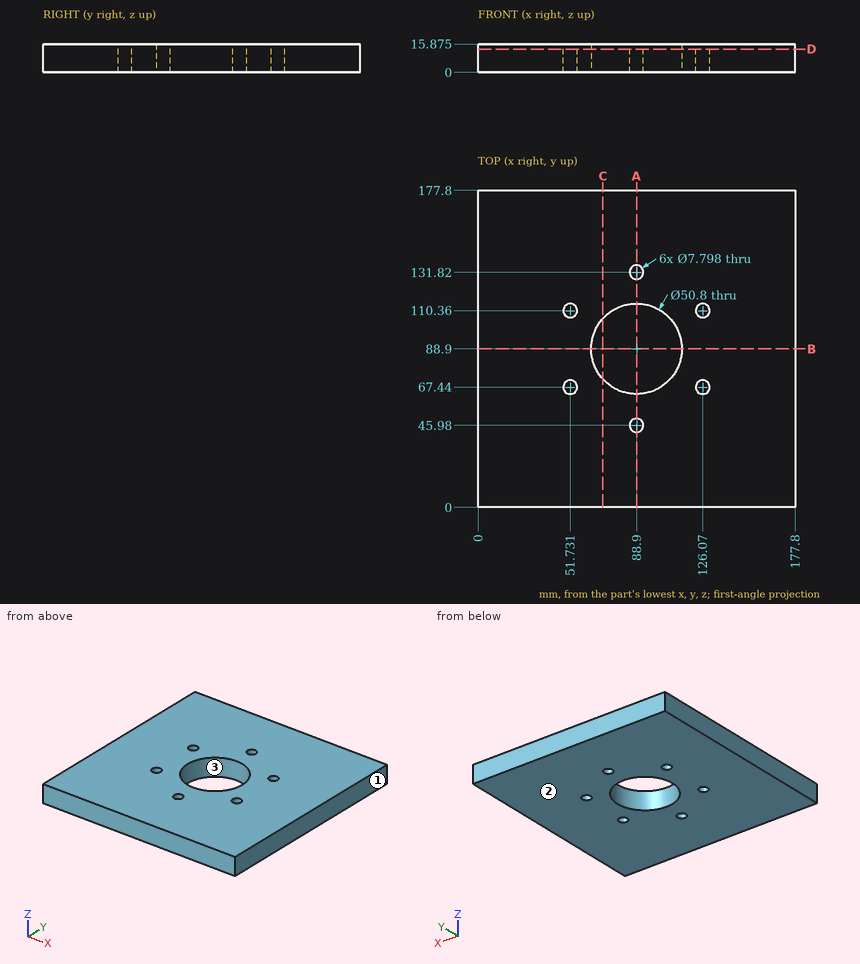
Geometry: see drawing. Coordinates: mm, zero at the bounding-box minimum. Round coordinates to 2 decimals unless told otherwise and drop trailing zeros. Loops run counter-clockwise (first coordinate to the right, second up) from the corner with the lowest first, then second, coordinate; pieces in that order, holes last. Notation, with made-up numbers: M 21.25,46.25 L 32.25,46.25 A10 ccw 32.25,64.25 Z; hole C 63.5,14 d10. An arc over 180 degrees is marked long. Use a Markdown table: item, result. Add a question column.
1. Contact query for flat-ended pins moving along their axis: pin 1 (10 mm diameter, centred on x = 126, y = 121, fed in from -Z); pin 2 (6 mm diameter, centred on x = 88.9, y = 45.98, fed in from +Z). Output: stop coordinate, or through.
2. Ray query, line 1 along X through (y, z) = (88.9, 11); line 2 along Y through (x, z) = (51, 9.5). Return the intervals inside material, ascending. Write a range as [from, to].
3. Pull-direction query (X, two-part tool) for the marked faces 1, 2 and 3; classes: +X half, -X half, draft (parallel to the pull), parting line (faces both ways), or undercut.
4. Cut plane A-A, the plane x = 88.9. Output: boundary loops of the cut face in (y, z) (1 decimal).
5. Cut plane D-D, the plane z = 13. Output: boundary loops of the cut face in (x, y), and give its area (3 significant figures).
6. Cut plane B-B, the plane y = 88.9. Output: boundary loops of the cut face in (x, z) (1 decimal), and give its area (3 significant figures).
7. Cut plane C-C, the plane x = 70. Output: boundary loops of the cut face in (y, z) (1 decimal).
Solution:
| question | item | result |
|---|---|---|
| 1 | pin 1 | stops at z = 0 |
| 1 | pin 2 | passes through |
| 2 | line 1 | x = [0, 63.5], [114.3, 177.8] |
| 2 | line 2 | y = [0, 63.61], [71.27, 106.53], [114.19, 177.8] |
| 3 | face 1 | +X half |
| 3 | face 2 | draft |
| 3 | face 3 | undercut |
| 4 | outline | M 0,0 L 42.1,0 L 42.1,15.9 L 0,15.9 Z; M 49.9,0 L 63.5,0 L 63.5,15.9 L 49.9,15.9 Z; M 114.3,0 L 127.9,0 L 127.9,15.9 L 114.3,15.9 Z; M 135.7,0 L 177.8,0 L 177.8,15.9 L 135.7,15.9 Z |
| 5 | outline | M 0,0 L 177.8,0 L 177.8,177.8 L 0,177.8 Z; hole C 51.73,67.44 d7.8; hole C 51.73,110.36 d7.8; hole C 88.9,88.9 d50.8; hole C 88.9,45.98 d7.8; hole C 88.9,131.82 d7.8; hole C 126.07,67.44 d7.8; hole C 126.07,110.36 d7.8 |
| 5 | area | 29,300 mm2 |
| 6 | outline | M 0,0 L 63.5,0 L 63.5,15.9 L 0,15.9 Z; M 114.3,0 L 177.8,0 L 177.8,15.9 L 114.3,15.9 Z |
| 6 | area | 2,020 mm2 |
| 7 | outline | M 0,0 L 71.9,0 L 71.9,15.9 L 0,15.9 Z; M 105.9,0 L 177.8,0 L 177.8,15.9 L 105.9,15.9 Z |
